CAD build for the part. Positions are in the model's coordinates, mm. A direction names the side the tool comes from. Round coordinates to 2 decimals unless told otherwise and drop trailing zeros. Order: outer loops, then holes, each group sorted by start corner. A loop starts at its lowest first (then second) coordinate and runs counter-clockwise, first axis right, second up.
```python
from build123d import *

# Parameters (mm, degrees)
SKETCH_1_W                        = 72.5
SKETCH_1_H                        = 22.1
SKETCH_1_R                        = 2.25
EXTRUDE_1_DEPTH                   = 17.2
SKETCH_2_W                        = 7.85
SKETCH_2_H                        = 22.1
CUT_EXTRUDE_1_DEPTH               = 7.2
SKETCH_3_W                        = 7.85
SKETCH_3_H                        = 3.3
CUT_EXTRUDE_2_DEPTH               = 2.1
SKETCH_4_R                        = 1.75
CUT_EXTRUDE_3_DEPTH               = 5
PATTERN_LINEAR_1_COUNT            = 6
PATTERN_LINEAR_1_PITCH            = 9
PATTERN_LINEAR_1_COPY_1_SKETCH_W  = 7.85
PATTERN_LINEAR_1_COPY_1_SKETCH_H  = 3.3
PATTERN_LINEAR_1_COPY_1_DEPTH     = 2.1
PATTERN_LINEAR_1_COPY_2_SKETCH_W  = 7.85
PATTERN_LINEAR_1_COPY_2_SKETCH_H  = 3.3
PATTERN_LINEAR_1_COPY_2_DEPTH     = 2.1
PATTERN_LINEAR_1_COPY_3_SKETCH_W  = 7.85
PATTERN_LINEAR_1_COPY_3_SKETCH_H  = 3.3
PATTERN_LINEAR_1_COPY_3_DEPTH     = 2.1
PATTERN_LINEAR_1_COPY_4_SKETCH_W  = 7.85
PATTERN_LINEAR_1_COPY_4_SKETCH_H  = 3.3
PATTERN_LINEAR_1_COPY_4_DEPTH     = 2.1
PATTERN_LINEAR_1_COPY_5_SKETCH_W  = 7.85
PATTERN_LINEAR_1_COPY_5_SKETCH_H  = 3.3
PATTERN_LINEAR_1_COPY_5_DEPTH     = 2.1
PATTERN_LINEAR_1_COPY_6_SKETCH_R  = 1.75
PATTERN_LINEAR_1_COPY_6_DEPTH     = 5
PATTERN_LINEAR_1_COPY_7_SKETCH_R  = 1.75
PATTERN_LINEAR_1_COPY_7_DEPTH     = 5
PATTERN_LINEAR_1_COPY_8_SKETCH_R  = 1.75
PATTERN_LINEAR_1_COPY_8_DEPTH     = 5
PATTERN_LINEAR_1_COPY_9_SKETCH_R  = 1.75
PATTERN_LINEAR_1_COPY_9_DEPTH     = 5
PATTERN_LINEAR_1_COPY_10_SKETCH_R = 1.75
PATTERN_LINEAR_1_COPY_10_DEPTH    = 5


with BuildPart() as part:
    # Sketch 1 → Extrude 1 (new body)
    with BuildSketch(Plane(origin=(0, 0, 0), x_dir=(1, 0, 0), z_dir=(0, 1, 0))):
        Rectangle(SKETCH_1_W, SKETCH_1_H)
        with Locations(Location((31, 0, 0), (0, 0, 90))):
            Circle(SKETCH_1_R, mode=Mode.SUBTRACT)
        with Locations(Location((-31, 0, 0), (0, 0, 90))):
            Circle(SKETCH_1_R, mode=Mode.SUBTRACT)
    extrude(amount=EXTRUDE_1_DEPTH)

    # Sketch 2 → Cut-Extrude 1 (cut)
    with BuildSketch(Plane(origin=(0, 17.2, 0), x_dir=(1, 0, 0), z_dir=(0, 1, 0))):
        with Locations((22.5, 0)):
            Rectangle(SKETCH_2_W, SKETCH_2_H)
    cut_extrude_1 = extrude(amount=-CUT_EXTRUDE_1_DEPTH, mode=Mode.SUBTRACT)

    # Sketch 3 → Cut-Extrude 2 (cut)
    with BuildSketch(Plane(origin=(0, 10, 0), x_dir=(1, 0, 0), z_dir=(0, 1, 0))):
        with Locations((22.5, 9.4)):
            Rectangle(SKETCH_3_W, SKETCH_3_H)
    cut_extrude_2 = extrude(amount=-CUT_EXTRUDE_2_DEPTH, mode=Mode.SUBTRACT)

    # Sketch 4 → Cut-Extrude 3 (cut)
    with BuildSketch(Plane(origin=(0, 10, 0), x_dir=(1, 0, 0), z_dir=(0, 1, 0))):
        with Locations(Location((22.5, 4, 0), (0, 0, 270))):
            Circle(SKETCH_4_R)
    cut_extrude_3 = extrude(amount=-CUT_EXTRUDE_3_DEPTH, mode=Mode.SUBTRACT)

    # Mirror 1: Cut-Extrude 2, Cut-Extrude 3 across plane
    add(cut_extrude_2.mirror(Plane.XY), mode=Mode.SUBTRACT)
    add(cut_extrude_3.mirror(Plane.XY), mode=Mode.SUBTRACT)

    # Pattern Linear 1: Cut-Extrude 1, Cut-Extrude 2, Cut-Extrude 3 ×6
    with Locations(*[(-i * PATTERN_LINEAR_1_PITCH, 0, 0) for i in range(1, PATTERN_LINEAR_1_COUNT)]):
        add(cut_extrude_1, mode=Mode.SUBTRACT)
        add(cut_extrude_2, mode=Mode.SUBTRACT)
        add(cut_extrude_3, mode=Mode.SUBTRACT)

    # Pattern Linear 1 copy 1 sketch → Pattern Linear 1 copy 1 (cut)
    with BuildSketch(Plane(origin=(-9, 10, 0), x_dir=(1, 0, 0), z_dir=(0, 1, 0))):
        with Locations((22.5, -9.4)):
            Rectangle(PATTERN_LINEAR_1_COPY_1_SKETCH_W, PATTERN_LINEAR_1_COPY_1_SKETCH_H)
    extrude(amount=-PATTERN_LINEAR_1_COPY_1_DEPTH, mode=Mode.SUBTRACT)

    # Pattern Linear 1 copy 2 sketch → Pattern Linear 1 copy 2 (cut)
    with BuildSketch(Plane(origin=(-18, 10, 0), x_dir=(1, 0, 0), z_dir=(0, 1, 0))):
        with Locations((22.5, -9.4)):
            Rectangle(PATTERN_LINEAR_1_COPY_2_SKETCH_W, PATTERN_LINEAR_1_COPY_2_SKETCH_H)
    extrude(amount=-PATTERN_LINEAR_1_COPY_2_DEPTH, mode=Mode.SUBTRACT)

    # Pattern Linear 1 copy 3 sketch → Pattern Linear 1 copy 3 (cut)
    with BuildSketch(Plane(origin=(-27, 10, 0), x_dir=(1, 0, 0), z_dir=(0, 1, 0))):
        with Locations((22.5, -9.4)):
            Rectangle(PATTERN_LINEAR_1_COPY_3_SKETCH_W, PATTERN_LINEAR_1_COPY_3_SKETCH_H)
    extrude(amount=-PATTERN_LINEAR_1_COPY_3_DEPTH, mode=Mode.SUBTRACT)

    # Pattern Linear 1 copy 4 sketch → Pattern Linear 1 copy 4 (cut)
    with BuildSketch(Plane(origin=(-36, 10, 0), x_dir=(1, 0, 0), z_dir=(0, 1, 0))):
        with Locations((22.5, -9.4)):
            Rectangle(PATTERN_LINEAR_1_COPY_4_SKETCH_W, PATTERN_LINEAR_1_COPY_4_SKETCH_H)
    extrude(amount=-PATTERN_LINEAR_1_COPY_4_DEPTH, mode=Mode.SUBTRACT)

    # Pattern Linear 1 copy 5 sketch → Pattern Linear 1 copy 5 (cut)
    with BuildSketch(Plane(origin=(-45, 10, 0), x_dir=(1, 0, 0), z_dir=(0, 1, 0))):
        with Locations((22.5, -9.4)):
            Rectangle(PATTERN_LINEAR_1_COPY_5_SKETCH_W, PATTERN_LINEAR_1_COPY_5_SKETCH_H)
    extrude(amount=-PATTERN_LINEAR_1_COPY_5_DEPTH, mode=Mode.SUBTRACT)

    # Pattern Linear 1 copy 6 sketch → Pattern Linear 1 copy 6 (cut)
    with BuildSketch(Plane(origin=(-9, 10, 0), x_dir=(1, 0, 0), z_dir=(0, 1, 0))):
        with Locations((22.5, -4)):
            Circle(PATTERN_LINEAR_1_COPY_6_SKETCH_R)
    extrude(amount=-PATTERN_LINEAR_1_COPY_6_DEPTH, mode=Mode.SUBTRACT)

    # Pattern Linear 1 copy 7 sketch → Pattern Linear 1 copy 7 (cut)
    with BuildSketch(Plane(origin=(-18, 10, 0), x_dir=(1, 0, 0), z_dir=(0, 1, 0))):
        with Locations((22.5, -4)):
            Circle(PATTERN_LINEAR_1_COPY_7_SKETCH_R)
    extrude(amount=-PATTERN_LINEAR_1_COPY_7_DEPTH, mode=Mode.SUBTRACT)

    # Pattern Linear 1 copy 8 sketch → Pattern Linear 1 copy 8 (cut)
    with BuildSketch(Plane(origin=(-27, 10, 0), x_dir=(1, 0, 0), z_dir=(0, 1, 0))):
        with Locations((22.5, -4)):
            Circle(PATTERN_LINEAR_1_COPY_8_SKETCH_R)
    extrude(amount=-PATTERN_LINEAR_1_COPY_8_DEPTH, mode=Mode.SUBTRACT)

    # Pattern Linear 1 copy 9 sketch → Pattern Linear 1 copy 9 (cut)
    with BuildSketch(Plane(origin=(-36, 10, 0), x_dir=(1, 0, 0), z_dir=(0, 1, 0))):
        with Locations((22.5, -4)):
            Circle(PATTERN_LINEAR_1_COPY_9_SKETCH_R)
    extrude(amount=-PATTERN_LINEAR_1_COPY_9_DEPTH, mode=Mode.SUBTRACT)

    # Pattern Linear 1 copy 10 sketch → Pattern Linear 1 copy 10 (cut)
    with BuildSketch(Plane(origin=(-45, 10, 0), x_dir=(1, 0, 0), z_dir=(0, 1, 0))):
        with Locations((22.5, -4)):
            Circle(PATTERN_LINEAR_1_COPY_10_SKETCH_R)
    extrude(amount=-PATTERN_LINEAR_1_COPY_10_DEPTH, mode=Mode.SUBTRACT)


solid = part.part
```
1. Cut at D-D, the plane z = 6.5. Write the cut outline in (x, y) (3 decimals).
2. Cut at A-A, the plane y = 14.5. Give the number of separate pieces and of enclosed holes in the cut face, and give its area (3 significant figures).
3. Tool access for faces 4 (the face through (22, 7.9, 9)), 5 (the face through (22, 7.9, -9)), 6 (the face through (-23, 10, 0)): list every direction of +Z, -Z, +X, -X, +Y, -Y with a clear straight run to the whole face (end or side of a thin tool).
4. Drill centre lines: line 1 (X direction, y = 9.5, z = 0); line 2 (Y direction, x = 3, z = 2.5); line 3 (Z direction, x = -5, y = 7.5). Where is each one in solid material? Low to high.
5. Cut at C-C, the plane x = -7. Write the cut outline in (y, z), and give its area (3 significant figures).
6. Mould opens along X. For faces 1 (the face through (9.575, 14, 0)), 2 (the face through (-1, 7, 11.05)), 3 (the face through (-11.765, 7.535, -4.228)) say: released by +X, released by -X, zero draft, split by the parting line, or undercut.
7. Pin check, flat tips, straight feed: P1, Ø2.5, axis at x = -23, z = -9.5, coming from the +Y side; P2, Ø6.5, axis at x = 22, z = -3, coming from the +Y side; P3, Ø1, axis at x = 23, z = 4.5, coming from the +Y side. Stop position of each tip, or through.
8. Cut at B-B, the plane x = -31. Write the cut outline in (y, z), and give its area (3 significant figures).
Outcome:
1. outline: (-36.25, 0) - (36.25, 0) - (36.25, 17.2) - (26.425, 17.2) - (26.425, 10) - (18.575, 10) - (18.575, 17.2) - (17.425, 17.2) - (17.425, 10) - (9.575, 10) - (9.575, 17.2) - (8.425, 17.2) - (8.425, 10) - (0.575, 10) - (0.575, 17.2) - (-0.575, 17.2) - (-0.575, 10) - (-8.425, 10) - (-8.425, 17.2) - (-9.575, 17.2) - (-9.575, 10) - (-17.425, 10) - (-17.425, 17.2) - (-18.575, 17.2) - (-18.575, 10) - (-26.425, 10) - (-26.425, 17.2) - (-36.25, 17.2) - close
2. separate pieces: 7
2. enclosed holes: 2
2. area: 530 mm2
3. face 4: +Z, +Y
3. face 5: -Z, +Y
3. face 6: +Z, -Z, +Y
4. line 1: x = -36.25 to -33.25, -28.75 to 28.75, 33.25 to 36.25
4. line 2: y = 0 to 10
4. line 3: z = -11.05 to -5.68, -2.32 to 2.32, 5.68 to 11.05
5. outline: (0, -11.05) - (7.9, -11.05) - (7.9, -7.75) - (10, -7.75) - (10, 7.75) - (7.9, 7.75) - (7.9, 11.05) - (0, 11.05) - close
5. area: 207 mm2
6. face 1: undercut
6. face 2: zero draft
6. face 3: undercut
7. P1: stops at y = 7.9
7. P2: stops at y = 10
7. P3: stops at y = 5
8. outline: (0, -11.05) - (17.2, -11.05) - (17.2, -2.25) - (0, -2.25) - close; (0, 2.25) - (17.2, 2.25) - (17.2, 11.05) - (0, 11.05) - close
8. area: 303 mm2
